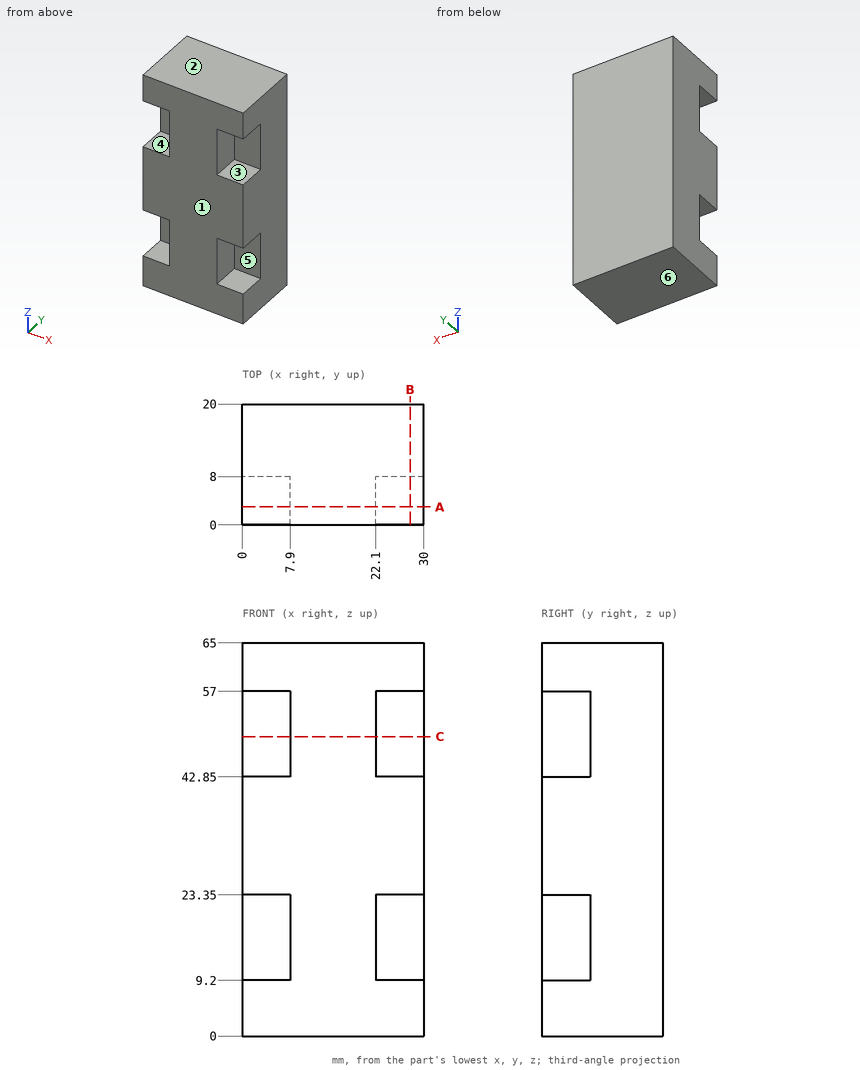
Job drawing, mm, ordinate dimensions from the low corner. One solid piece. A direction names the side the tool comes from. Coordinates: 2 decimals unless noted, no trailing zeros. Write each loop counter-clockwise with the first axis right and the second up, starting at its lowest first coordinate (ties: lowest second). Pieces come first, ordered by that corner, then holes. Notation, with made-up numbers: M 73,50.25 L 121,50.25 A26 ccw 121,67.25 Z; hole C -15.5,51.25 d6. An arc over 180 degrees is marked long. Answer as a JSON object with one key per item and string values. Group by question number.
1) Saw through at A-A (y = 3). Write the cut outline in (x, z).
2) Tool access for the marked faces 4, 5 and 6: list every direction of +Z, -Z, +X, -X, +Y, -Y with a clear straight run to the whole face (end or side of a thin tool).
3) Wall check: line 1 (Z direction, x = 27.25, y = 1); line 2 (X direction, y = 4.25, z = 14); line 3 (Y direction, x = 22.25, z = 13). Give the ranges that are in metal, low to high. Write a range as from..to.
4) Saw through at C-C (z = 49.5). Write the cut outline in (x, y).
5) Mould opens along Z. For the marked faces 1, 2 and 3 say: +Z half, -Z half, draft (parallel to the pull), parting line (faces both ways), or undercut.
6) Pin check, flat tips, straight feed: pin 1 Ø2.5 at (x, z) = (3, 47) entering from -Y; pin 2 Ø4 at (y, z) = (2, 48.5) entering from +X; pin 3 Ø6.5 at (y, z) = (3.5, 16.5) entering from -X. Stop position of each tip, or through.
7) Saw through at B-B (x = 27.75). Write the cut outline in (y, z).
Values follow:
{
 "1": {"outline": "M 0,0 L 30,0 L 30,9.2 L 22.1,9.2 L 22.1,23.35 L 30,23.35 L 30,42.85 L 22.1,42.85 L 22.1,57 L 30,57 L 30,65 L 0,65 L 0,57 L 7.9,57 L 7.9,42.85 L 0,42.85 L 0,23.35 L 7.9,23.35 L 7.9,9.2 L 0,9.2 Z"},
 "2": {"face 4": "-X, -Y", "face 5": "+X, -Y", "face 6": "-Z, +X, -X, +Y, -Y"},
 "3": {"line 1": "z = 0..9.2, 23.35..42.85, 57..65", "line 2": "x = 7.9..22.1", "line 3": "y = 8..20"},
 "4": {"outline": "M 0,8 L 7.9,8 L 7.9,0 L 22.1,0 L 22.1,8 L 30,8 L 30,20 L 0,20 Z"},
 "5": {"face 1": "draft", "face 2": "+Z half", "face 3": "undercut"},
 "6": {"pin 1": "stops at y = 8", "pin 2": "stops at x = 22.1", "pin 3": "stops at x = 7.9"},
 "7": {"outline": "M 0,0 L 20,0 L 20,65 L 0,65 L 0,57 L 8,57 L 8,42.85 L 0,42.85 L 0,23.35 L 8,23.35 L 8,9.2 L 0,9.2 Z"}
}
